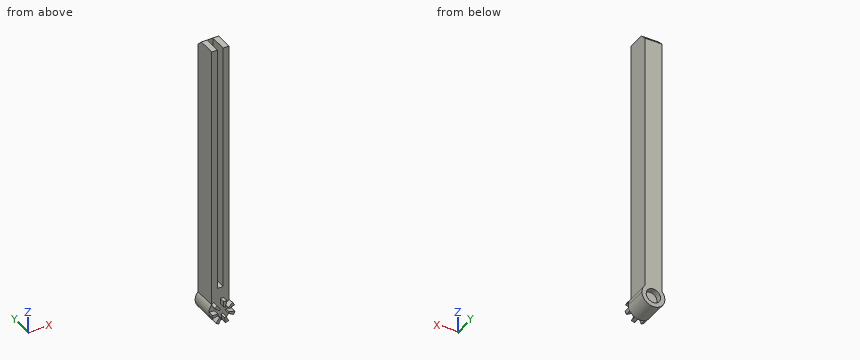
from build123d import *

# Parameters (mm, degrees)
F1_DEPTH = 12.7
F2_W     = 3.175
F2_H     = 9.525
F3_DEPTH = 139.7
F5_DEPTH = 3.175
F6_R     = 3.96875
F7_DEPTH = 3.175
F8_SIZE  = 3.17499


# Not quite as in the source:
# - a fillet or chamfer is up to 0.001 mm smaller than in the source, because OpenCascade refuses the exact size


with BuildPart() as f1:
    # F0 (on Front) → F1 (new body)
    with BuildSketch(Plane.XZ):
        with BuildLine():
            Line((0, 152.4), (0, 4.2001302063))
            ThreePointArc((0, 4.2001302063), (4.7625, 6.35), (9.525, 4.2001302063))
            Line((9.525, 4.2001302063), (9.525, 152.4))
            Line((9.525, 152.4), (0, 152.4))
        make_face()
        with BuildLine():
            Line((0, 4.2001302063), (0, 0))
            Line((0, 0), (9.525, 0))
            Line((9.525, 0), (9.525, 4.2001302063))
            ThreePointArc((9.525, 4.2001302063), (4.7625, 6.35), (0, 4.2001302063))
        make_face()
        with BuildLine():
            Line((9.525, 0), (0, 0))
            Line((0, 0), (0, 4.2001302063))
            ThreePointArc((0, 4.2001302063), (2.5174359697, -5.9398811015), (11.1125, 0))
            ThreePointArc((11.1125, 0), (10.7023811015, 2.2450640303), (9.525, 4.2001302063))
            Line((9.525, 4.2001302063), (9.525, 0))
        make_face()
    extrude(amount=F1_DEPTH)

    # F2 (on face) → F3 (cut)
    with BuildSketch(Plane.XY.offset(152.4)):
        with Locations((4.7625, -7.9375)):
            Rectangle(F2_W, F2_H)
    extrude(amount=-F3_DEPTH, mode=Mode.SUBTRACT)

    # F4 (on face) → F5 (join)
    with BuildSketch(Plane.XZ.offset(12.7)):
        with BuildLine():
            Line((5.2357091951, -3.1395378733), (5.7089183902, -6.2790757465))
            ThreePointArc((5.7089183902, -6.2790757465), (6.6341953575, -6.0678873167), (7.5176617434, -5.7211523112))
            Line((7.5176617434, -5.7211523112), (6.1400808717, -2.8605761556))
            ThreePointArc((6.1400808717, -2.8605761556), (5.6983476788, -3.0339436584), (5.2357091951, -3.1395378733))
        make_face()
        with BuildLine():
            Line((2.6029515576, -2.3274396931), (0.4434031152, -4.6548793861))
            ThreePointArc((0.4434031152, -4.6548793861), (1.1854176313, -5.2466162169), (2.0073382566, -5.7211523112))
            Line((2.0073382566, -5.7211523112), (3.3849191283, -2.8605761556))
            ThreePointArc((3.3849191283, -2.8605761556), (2.9739588156, -2.6233081085), (2.6029515576, -2.3274396931))
        make_face()
        with BuildLine():
            Line((1.5963779439, 0.2372680471), (-1.5697441121, 0.4745360943))
            ThreePointArc((-1.5697441121, 0.4745360943), (-1.5697441121, -0.4745360943), (-1.4282922424, -1.4130079306))
            Line((-1.4282922424, -1.4130079306), (1.6671038788, -0.7065039653))
            ThreePointArc((1.6671038788, -0.7065039653), (1.5963779439, -0.2372680471), (1.5963779439, 0.2372680471))
        make_face()
        with BuildLine():
            ThreePointArc((2.2801850432, 1.9795801209), (2.6029515576, 2.3274396931), (2.9739588156, 2.6233081085))
            Line((2.9739588156, 2.6233081085), (1.1854176313, 5.2466162169))
            ThreePointArc((1.1854176313, 5.2466162169), (0.5600076724, 4.760415763), (0, 4.2001302063))
            ThreePointArc((0, 4.2001302063), (-0.1025571138, 4.080896872), (-0.2021299137, 3.9591602418))
            Line((-0.2021299137, 3.9591602418), (2.2801850432, 1.9795801209))
        make_face()
        with BuildLine():
            Line((4.7625, 6.35), (4.7625, 3.175))
            ThreePointArc((4.7625, 3.175), (5.2357091951, 3.1395378733), (5.6983476788, 3.0339436584))
            Line((5.6983476788, 3.0339436584), (6.6341953575, 6.0678873167))
            ThreePointArc((6.6341953575, 6.0678873167), (5.7089183902, 6.2790757465), (4.7625, 6.35))
        make_face()
        with BuildLine():
            ThreePointArc((10.6735483039, 2.3199155047), (10.261761314, 3.175), (9.7271299137, 3.9591602418))
            Line((9.7271299137, 3.9591602418), (7.2448149568, 1.9795801209))
            ThreePointArc((7.2448149568, 1.9795801209), (7.512130657, 1.5875), (7.7180241519, 1.1599577524))
            Line((7.7180241519, 1.1599577524), (10.6735483039, 2.3199155047))
        make_face()
        with BuildLine():
            Line((7.512130657, -1.5875), (10.261761314, -3.175))
            ThreePointArc((10.261761314, -3.175), (10.6735483039, -2.3199155047), (10.9532922424, -1.4130079306))
            Line((10.9532922424, -1.4130079306), (7.8578961212, -0.7065039653))
            ThreePointArc((7.8578961212, -0.7065039653), (7.7180241519, -1.1599577524), (7.512130657, -1.5875))
        make_face()
    extrude(amount=F5_DEPTH)

    # F6 (on face) → F7 (cut)
    with BuildSketch(Plane(origin=(0, 0, 0), x_dir=(-1, 0, 0), z_dir=(0, 1, 0))):
        with Locations((-4.7625, 0)):
            Circle(F6_R)
    extrude(amount=-F7_DEPTH, mode=Mode.SUBTRACT)

    # F8 (size 3.175 in the source; OpenCascade refuses exactly that, so slightly less here)
    f8_edges = [f1.edges().sort_by_distance(p)[0] for p in [
        (4.7625, 0, 152.4),
    ]]
    chamfer(f8_edges, length=F8_SIZE)


solid = f1.part
Could you check a few things on this model? Use its own coordinates, in mm. Round coordinates to 2 decimals unless told otherwise and drop trailing zeros. Order: outer loops, then holes, each group sorted by start corner. A loop starts at its lowest first (then second) coordinate and runs counter-clockwise, first axis right, second up. Notation, with made-up numbers: M 71.5,38 L 99.5,38 A11 cw 99.5,54 Z; hole C 55.25,-25.5 d8. An arc over 180 degrees is marked long. One line per item, written item: value.
(1) I'm going to push flat-ended pins straight in: P1, Ø3, axis at x = 7, y = -13.5, coming from the +Z side; P2, Ø5, axis at y = -8.5, z = 115, coming from the -X side; P3, Ø3, axis at x = 0, y = -14.5, coming from the +Z side; P4, Ø3, axis at x = 5, y = -13.5, coming from the +Z side. Where does each tip first touch, or does it pass through?
Ans:
P1: stops at z = 152.4
P2: stops at x = 0
P3: stops at z = 5.25
P4: stops at z = 12.7
(2) I need wall thicknesses on line 1 along X through (y, z) = (-5, 56) (3 decimals); line 2 along Z through (x, y) = (1, -15); line 3 along Y through (x, z) = (1, 57). Which ranges of each line are inside material? Lowest first, please. Write a range as from..to.
Ans:
line 1: x = 0..3.175, 6.35..9.525
line 2: z = -5.12..-4.06, -0.86..0.28, 3..5.12
line 3: y = -12.7..0
(3) Imagine slicing it at A-A (y = -14). Count the separate pieces of the cut face and the enclosed holes in it, and give its area (3 significant figures).
Ans:
separate pieces: 7
enclosed holes: 0
area: 31.7 mm^2
(4) Imagine slicing it at B-B (z = 112). Write out the boundary of the cut face in (x, y) (3 decimals), and give its area (3 significant figures).
Ans:
outline: M 0,-12.7 L 3.175,-12.7 L 3.175,-3.175 L 6.35,-3.175 L 6.35,-12.7 L 9.525,-12.7 L 9.525,0 L 0,0 Z
area: 90.7 mm^2
